Design review of the part shown in the three views and the two pictorial views. Dimensions are in mm from the part's minimum x, y and z. Coordinates: 2 decimals unless noted, no trailing zeros. Loops run counter-clockwise (first coordinate to the right, second up) from the corner with the lowest first, then second, coordinate; pieces in that order, holes last. Notation, with made-up numbers: (84.25, 79.5) -> (143.25, 79.5) arc R18 cw to (143.25, 96.5) -> close; hole circle Ø4 at (13, -1.5). An arc over 180 degrees is marked (long way). Use CSV: the item, a comma, the result in double quotes.
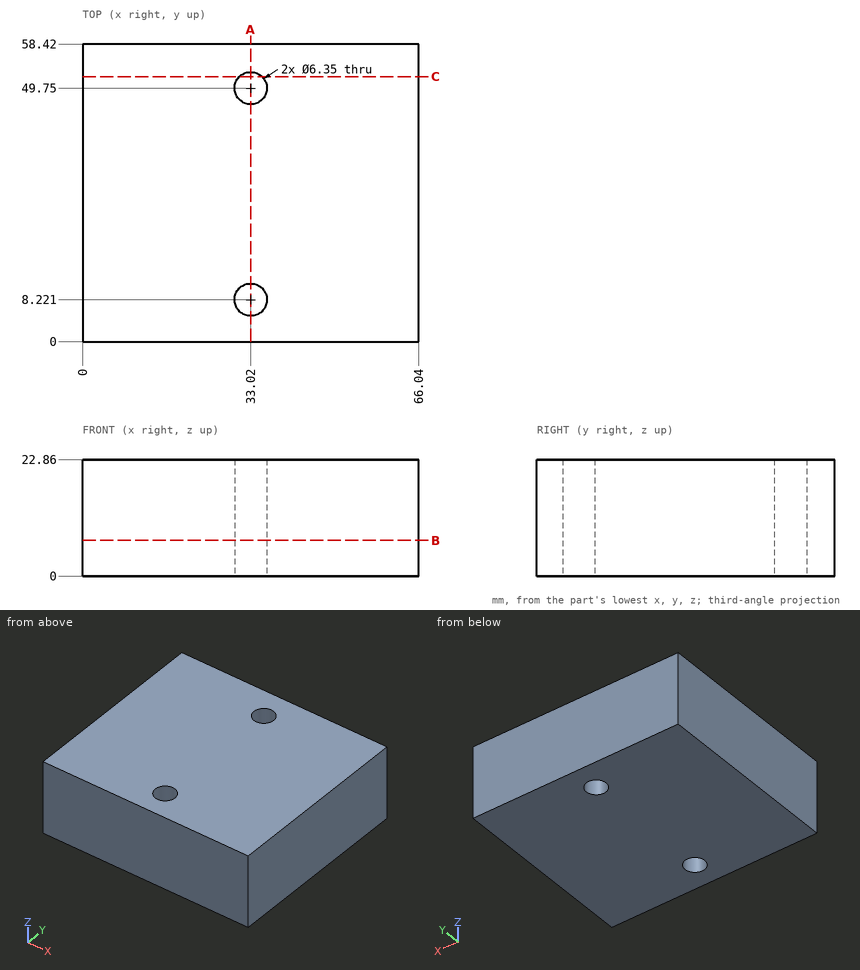
Item 1: Add section B-B (z = 7). Give the boundary of the cut face in (x, y) (3 decimals).
Checked values:
outline,"(0, 0) -> (66.04, 0) -> (66.04, 58.42) -> (0, 58.42) -> close; hole circle Ø6.35 at (33.02, 8.221); hole circle Ø6.35 at (33.02, 49.75)"
Item 2: Clearance check with flat-ended pins moving along their axes: pin 1 (10 mm diameter, centred on x = 26, z = 17.5, fed in from -Y); pin 2 (2 mm diameter, centred on x = 34.5, y = 7.5, fed in from +Z). State where each tip first meets the part, or that it passes through.
Checked values:
pin 1,"y = 0"
pin 2,"through"
Item 3: Add section A-A (x = 33.02). Give the boundary of the cut face in (y, z) (3 decimals).
Checked values:
outline,"(0, 0) -> (5.046, 0) -> (5.046, 22.86) -> (0, 22.86) -> close; (11.396, 0) -> (46.575, 0) -> (46.575, 22.86) -> (11.396, 22.86) -> close; (52.925, 0) -> (58.42, 0) -> (58.42, 22.86) -> (52.925, 22.86) -> close"
Item 4: To check wall thickness, follow line 1 along Y through (x, z) = (33.02, 11.25) (3 decimals); line 2 along X through (y, z) = (51, 5.25). State the ranges of each line that lie inside material, in increasing order.
Checked values:
line 1,"0 to 5.046, 11.396 to 46.575, 52.925 to 58.42"
line 2,"0 to 30.1, 35.94 to 66.04"
Item 5: Add section C-C (y = 52). Give the boundary of the cut face in (x, z), then the cut area to 3 significant figures.
Checked values:
outline,"(0, 0) -> (30.78, 0) -> (30.78, 22.86) -> (0, 22.86) -> close; (35.26, 0) -> (66.04, 0) -> (66.04, 22.86) -> (35.26, 22.86) -> close"
area,"1,410 mm^2"
